from build123d import *

# Parameters (mm, degrees)
F1_DEPTH = 18
F2_R     = 2
F3_DEPTH = 6
F4_R     = 2
F5_R     = 6


with BuildPart() as f1:
    # F0 (on Front) → F1 (new body)
    with BuildSketch(Plane.XZ):
        with BuildLine():
            ThreePointArc((25.212652, -19.867868), (0, -32.1), (-25.212652, -19.867868))
            ThreePointArc((-25.212652, -19.867868), (-30.513321, 0.829972), (-21.663506, 20.276783))
            ThreePointArc((-21.663506, 20.276783), (-21.384271, 20.979731), (-21.677117, 21.677117))
            Line((-21.677117, 21.677117), (-22.384578, 22.384578))
            ThreePointArc((-22.384578, 22.384578), (-22.564076, 22.526959), (-22.77127, 22.624748))
            ThreePointArc((-22.77127, 22.624748), (-23.308835, 22.653609), (-23.783467, 22.399576))
            ThreePointArc((-23.783467, 22.399576), (-31.56023, 11.156534), (-34.29906, -2.236855))
            Line((-34.29906, -2.236855), (-34.29906, -35.098328))
            Line((-34.29906, -35.098328), (-52, -35.098328))
            Line((-52, -35.098328), (-52, -41.098328))
            Line((-52, -41.098328), (0, -41.098328))
            Line((0, -41.098328), (52, -41.098328))
            Line((52, -41.098328), (52, -35.098328))
            Line((52, -35.098328), (34.29906, -35.098328))
            Line((34.29906, -35.098328), (34.29906, -2.236855))
            ThreePointArc((34.29906, -2.236855), (31.56023, 11.156534), (23.783467, 22.399576))
            ThreePointArc((23.783467, 22.399576), (23.308835, 22.653609), (22.77127, 22.624748))
            ThreePointArc((22.77127, 22.624748), (22.564076, 22.526959), (22.384578, 22.384578))
            Line((22.384578, 22.384578), (21.677117, 21.677117))
            ThreePointArc((21.677117, 21.677117), (21.384271, 20.979731), (21.663506, 20.276783))
            ThreePointArc((21.663506, 20.276783), (30.513321, 0.829972), (25.212652, -19.867868))
        make_face()
    extrude(amount=F1_DEPTH)

    # F2 (on face) → F3 (cut, through all)
    with BuildSketch(Plane(origin=(0, 0, -41.098328), x_dir=(1, 0, 0), z_dir=(0, 0, -1))):
        with Locations((-45, 9)):
            Circle(F2_R)
        with Locations((45, 9)):
            Circle(F2_R)
    extrude(amount=-F3_DEPTH, mode=Mode.SUBTRACT)

    # F4
    f4_edges = [f1.edges().sort_by_distance(p)[0] for p in [
        (-52, 0, -38.098328),
        (-52, -18, -38.098328),
        (52, -18, -38.098328),
        (52, 0, -38.098328),
    ]]
    fillet(f4_edges, radius=F4_R)

    # F5
    f5_edges = [f1.edges().sort_by_distance(p)[0] for p in [
        (-34.29906, -9, -35.098328),
        (34.29906, -9, -35.098328),
    ]]
    fillet(f5_edges, radius=F5_R)


solid = f1.part
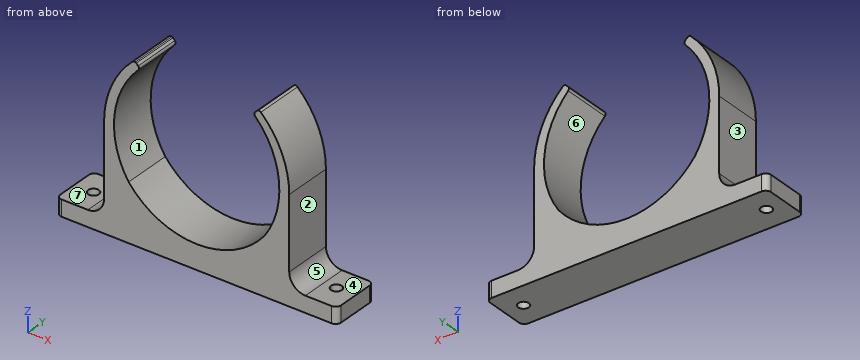
Build history of the part. All positions in model axes, mm. Face numbers are marked on the shaded views. A direction names the side the tool comes from. Round coordinates to 2 decimals unless told otherwise and drop trailing zeros. Write each loop counter-clockwise with the first axis right and the second up, starting at its lowest first coordinate (ties: lowest second). Pieces come first, ordered by that corner, then holes. Notation, with made-up numbers: (13, 78) - (28, 78) arc R22 cw to (28, 91) - close; hole circle Ø8 at (44, -20). An arc over 180 degrees is marked (long way). One line per question, with ' | ' between items.
1. Band-saw the part on B-B, the plane x = -45. Write the cut outline in (y, z), and give its area (3 significant figures).
Results are:
outline: (-18, -41.1) - (-11, -41.1) - (-11, -35.1) - (-18, -35.1) - close; (-7, -41.1) - (0, -41.1) - (0, -35.1) - (-7, -35.1) - close | area: 84.0 mm^2
2. Band-saw the part on A-A, the plane y = -9. Give the number of separate pieces and of enclosed holes in the cut face, and give its area (3 significant figures).
Results are:
separate pieces: 3 | enclosed holes: 0 | area: 1,580 mm^2
3. Drop flat-ended pins along their axis: pin 1 Ø6 at (x, y) = (46.5, -7) entering from +Z; pin 2 Ø5.5 at (y, z) = (-11.5, -11) entering from +X; pin 3 Ø5.5 at (y, z) = (-7, -18.5) entering from -X. Give the stop position or say it passes through.
Results are:
pin 1: z = -35.1 | pin 2: x = 34.3 | pin 3: x = -34.3
4. Band-saw the part on C-C, the plane z = 11. Write the cut outline in (x, y), and give its area (3 significant figures).
Results are:
outline: (-31.63, -18) - (-27.89, -18) - (-27.89, 0) - (-31.63, 0) - close; (27.89, -18) - (31.63, -18) - (31.63, 0) - (27.89, 0) - close | area: 134 mm^2
5. Band-saw the part on D-D, the plane x = 36. Write the cut outline in (y, z), and give its area (3 significant figures).
Results are:
outline: (-18, -41.1) - (0, -41.1) - (0, -33.28) - (-18, -33.28) - close | area: 141 mm^2
6. Drill centre lines: line 1 along X through (y, z) = (-9, -36.9); line 2 along Y through (x, z) = (45, -39); line 3 along X through (y, z) = (-14.25, -13.5). Where is each one in solid material? Low to high. Write a range as from..to.
Results are:
line 1: -52..-47, -43..43, 47..52 | line 2: -18..-11, -7..0 | line 3: -34.3..-28.51, 28.51..34.3
7. Mould opens along X. For the marked faces 1, 2, 3 and 4 say: released by +X, released by -X, zero draft, split by the parting line, or undercut.
Results are:
face 1: undercut | face 2: released by +X | face 3: released by -X | face 4: zero draft
8. Tool access for the marked faces 5, 6 and 7: list every direction of +Z, -Z, +X, -X, +Y, -Y with a clear straight run to the whole face (end or side of a thin tool).
Results are:
face 5: +Z, +X, +Y, -Y | face 6: +Y, -Y | face 7: +Z, -X, +Y, -Y
